from build123d import *

# Parameters (mm, degrees)
SKETCH1_R           = 12.625
BOSS_EXTRUDE1_DEPTH = 5
SKETCH2_W           = 61.7
SKETCH2_H           = 59.5
SKETCH2_R           = 1.85
BOSS_EXTRUDE2_DEPTH = 5
FILLET1_RADIUS      = 29.75
FILLET1_LENGTH      = 5


with BuildPart() as part:
    # Sketch1 → Boss-Extrude1 (new body)
    with BuildSketch(Plane.XY):
        Polygon((-22.584548564, 28.565725374), (44.316590659, 32.204072605), (47.547660215, -27.208133124), (-19.353479009, -30.846480354), align=None)
        Circle(SKETCH1_R, mode=Mode.SUBTRACT)
    extrude(amount=BOSS_EXTRUDE1_DEPTH)

    # Sketch2 → Boss-Extrude2 (add)
    with BuildSketch(Plane(origin=(45.932125437, 2.49796974, 0), x_dir=(0, 0, -1), z_dir=(0.9985244660253657, 0.05430369001051772, 0))):
        with Locations((25.85, 0)):
            Rectangle(SKETCH2_W, SKETCH2_H)
        with Locations(Location((10.25, 19.75, 0), (0, 0, 90))):
            Circle(SKETCH2_R, mode=Mode.SUBTRACT)
        with Locations(Location((41.45, 19.75, 0), (0, 0, 90))):
            Circle(SKETCH2_R, mode=Mode.SUBTRACT)
        with Locations(Location((41.45, -19.75, 0), (0, 0, 90))):
            Circle(SKETCH2_R, mode=Mode.SUBTRACT)
        with Locations(Location((10.25, -19.75, 0), (0, 0, 90))):
            Circle(SKETCH2_R, mode=Mode.SUBTRACT)
    extrude(amount=BOSS_EXTRUDE2_DEPTH)

    # Fillet1: full round fillet: the end face becomes a half cylinder, R = half its width
    fillet1_face = Plane((-20.969013787, -1.14037749, 2.5), x_dir=(0, 0, -1), z_dir=(-0.998524466025, -0.054303690011, 0))  # on the end face: x along it, z out of the body
    fillet1_slab = fillet1_face.offset(-FILLET1_RADIUS / 2) * Box(FILLET1_LENGTH, 2 * FILLET1_RADIUS, FILLET1_RADIUS, mode=Mode.PRIVATE)  # the body's end, R deep
    fillet1_round = Plane((8.737089077, 0.475157288, 2.5), x_dir=(-0.998524466025, -0.054303690011, 0), z_dir=(0, 0, -1)) * Cylinder(FILLET1_RADIUS, FILLET1_LENGTH, mode=Mode.PRIVATE)  # its axis R under the face
    add(fillet1_slab - fillet1_round, mode=Mode.SUBTRACT)


solid = part.part
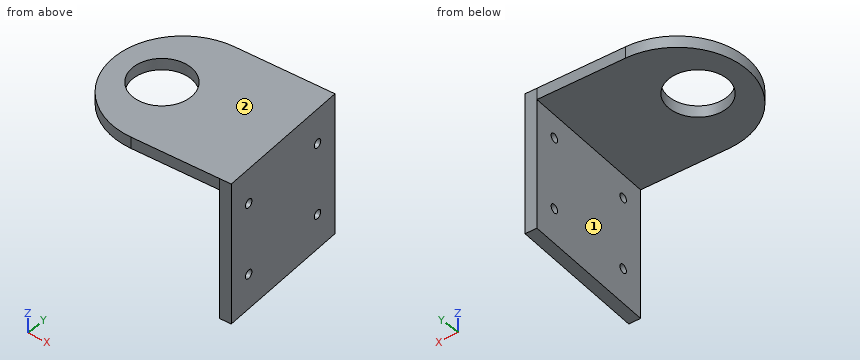
CAD build for the part. Positions are in the model's coordinates, mm. Face numbers are marked on the shaded views. A direction names the side the tool comes from. Round coordinates to 2 decimals unless told otherwise and drop trailing zeros. Write each loop counter-clockwise with the first axis right and the second up, starting at its lowest first coordinate (ties: lowest second). Pieces come first, ordered by that corner, then holes.
(1) Slice it at B-B, the plane y = -2. Write the cut outline in (x, z), and give its area (3 significant figures).
(2) Probe line 1 along Z through (x, y) = (35, 3); line 2 along Y through (x, z) = (0, 1.1) (3 decimals); line 3 along X through (y, z) = (-18, -26.5). List the from-to ranges inside material, lowest first.
(3) Slice it at A-A, the plane x = -6. Write the cut outline in (y, z).
(4) Slice it at C-C, the plane y = 9. Write the cut outline in (x, z), and give its area (3 significant figures).
(5) Slice it at D-D, the plane z = -25.5. Write the cut outline in (x, y), and give its area (4 significant figures).
(6) 3-axis set-ups, long thin cutter, end or side, ignore diameter. For the marked faces 1 and 2: which of +Z, -Z, +X, -X, +Y, -Y reach the whole face in a straight line?
(7) Drop flat-ended pins along their axis: P1, Ø5, axis at y = -13, z = -32, coming from the -X side; P2, Ø4, axis at y = -22.5, z = -28, coming from the -X side; P3, Ø12, axis at x = 3.5, y = -13.5, coming from the -Z side. Give the stop position or say it passes through.
From the geometry:
1. outline: (-20.91, 0) - (-12.47, 0) - (-12.47, 5) - (-20.91, 5) - close; (12.47, 0) - (46.18, 0) - (46.18, -56.7) - (51.18, -56.7) - (51.18, 5) - (12.47, 5) - close
1. area: 520 mm2
2. line 1: z = 0 to 5
2. line 2: y = -27.963 to -12.625, 12.625 to 28.913
2. line 3: x = 47.05 to 52.05
3. outline: (-25.37, 0) - (-11.11, 0) - (-11.11, 5) - (-25.37, 5) - close; (11.11, 0) - (26.32, 0) - (26.32, 5) - (11.11, 5) - close
4. outline: (-19.77, 0) - (-8.85, 0) - (-8.85, 5) - (-19.77, 5) - close; (8.85, 0) - (45.58, 0) - (45.58, -56.7) - (50.59, -56.7) - (50.59, 5) - (8.85, 5) - close
4. area: 547 mm2
5. outline: (44.32, 32.2) - (47.55, -27.21) - (52.54, -26.94) - (49.31, 32.48) - close
5. area: 297.5 mm2
6. face 1: -Z, -X, -Y
6. face 2: +Z, +X, -X, +Y, -Y
7. P1: stops at x = 46.64
7. P2: stops at x = 47.18
7. P3: stops at z = 0
